Model file for the job. Use its own axes, mm. A direction names the side the tool comes from. Round coordinates to 2 decimals unless told otherwise and drop trailing zeros. Loops run counter-clockwise (first coordinate to the right, second up) from the corner with the lowest first, then second, coordinate; pieces in that order, holes last. Notation, with made-up numbers: M 33.5,28.25 L 83.5,28.25 A22 ccw 83.5,51.25 Z; hole C -27,56 d9. An arc over 180 degrees is marked long. Use a Markdown table: item, result. Add a question column.
Item 1: Tool access for faces 1 (the cylindrical face through (-40.561, 40.755, 0.01)), 2 (the conical face through (-39.694, -39.869, -0.418)), 3 (the conical face through (-39.694, 39.869, 0.418)), 4 (the cylindrical face through (39.512, 39.683, -0.005)): list every direction of +Z, -Z, +X, -X, +Y, -Y with a clear straight run to the whole face (end or side of a thin tool).
Item 2: Saw through at C-C on z = 0.05. Write the cut outline in (x, y).
Item 3: Wall check: L1, parallel to Y at x = 17.5, z = 0.2; L2, parallel to X at y = 34.5, z = -0.05. Give the ranges that are in metal, low to high. Write a range as from..to.
Item 4: Two-plate mould, pull along Y, no slides. Class faces 5 (the cylindrical face through (40.755, 40.561, 0.01)), 6 (the cylindrical face through (39.683, -39.512, -0.005)), 7 (the cylindrical face through (40.561, -40.755, 0.01)): +Y half, -Y half, draft (parallel to the pull), parting line (faces both ways), or undercut.
Item 5: Saw through at A-A on y = 9.5. Write the cut outline in (x, z), then the cut area to 3 significant figures.
Autodesk Inventor part; units mm, degrees
ref_plane "YZ Plane" through (0, 0, 0) normal (1, 0, 0) x (0, 1, 0)
ref_plane "XZ Plane" through (0, 0, 0) normal (0, 1, 0) x (-1, 0, 0)
ref_plane "XY Plane" through (0, 0, 0) normal (0, 0, 1) x (1, 0, 0)
sketch "Sketch1" plane through (0, 0, 0) normal (0, 0, 1) x (1, 0, 0)
  line L0 (0, 0) -> (0, 7.5) construction
  line L1 (10, 0) -> (0, 0) construction
  line L2 (0, 0) -> (-10, 0) construction
  line L3 (0, 0) -> (-31.8198, 31.8198) construction
  circle A0 centre (0, 0) radius 45 construction
  line L4 (0, 0) -> (0, 45) construction
  line L5 (-31.8198, 31.8198) -> (-31.8198, -24.2384) construction
  line L6 (-31.8198, -24.2384) -> (-31.8198, -31.8198) construction
  line L7 (-31.8198, 31.8198) -> (24.2384, 31.8198) construction
  line L8 (24.2384, 31.8198) -> (31.8198, 31.8198) construction
  line L9 (31.8198, 31.8198) -> (31.8198, -31.8198) construction
  line L10 (31.8198, -31.8198) -> (-31.8198, -31.8198) construction
  line L11 (0, 0) -> (39.9999, 0) construction
  line L12 (0, 0) -> (0, -40) construction
  line L13 (-31.8198, 44.3198) -> (0, 44.3198)
  line L14 (-44.3198, 31.8198) -> (-44.3198, 0)
  line L15 (-44.3198, 0) -> (0, 0) construction
  arc A1 (-31.8198, 44.3198) -> (-44.3198, 31.8198) centre (-31.8198, 31.8198) ccw
  point P0 (0, 50)
  dimension "d6" = 90
  dimension "d7" = 45
  dimension "d15" = 12.5
sketch "Sketch2" plane through (0, 0, 0) normal (1, 0, 0) x (0, 1, 0)
  line L0 (44.3198, 0) -> (44.3198, 0.75)
  line L1 (44.3198, 0.75) -> (42.8198, 0.3481)
  line L2 (42.8198, 0.3481) -> (42.8198, 0)
  line L3 (44.3198, 0) -> (42.8198, 0) construction
  line L4 (44.3198, 0) -> (44.3198, -0.75)
  line L5 (44.3198, -0.75) -> (42.8198, -0.3481)
  line L6 (42.8198, -0.3481) -> (42.8198, 0)
  dimension "d16" = 0.75
  dimension "d17" = 15
  dimension "d18" = 1.5
sweep "Sweep1" add profiles "Sketch2" path "Sketch1"
mirror "Mirror1" about plane through (0, 43.6835, 0) normal (1, 0, 0) of "Sweep1"
mirror "Mirror2" about plane through (-44.3198, 0, 0) normal (0, -1, 0) of "Sweep1", "Mirror1"
properties part number "Belt"
Entries:
| question | item | result |
|---|---|---|
| 1 | face 1 | +Z, -Z, -X, +Y |
| 1 | face 2 | -Z |
| 1 | face 3 | +Z |
| 1 | face 4 | +Z, -Z |
| 2 | outline | M -44.32,-31.82 A12.5 ccw -31.82,-44.32 L 31.82,-44.32 A12.5 ccw 44.32,-31.82 L 44.32,31.82 A12.5 ccw 31.82,44.32 L -31.82,44.32 A12.5 ccw -44.32,31.82 Z; hole M -42.82,-31.82 A11 ccw -31.82,-42.82 L 31.82,-42.82 A11 ccw 42.82,-31.82 L 42.82,31.82 A11 ccw 31.82,42.82 L -31.82,42.82 A11 ccw -42.82,31.82 Z |
| 3 | L1 | -44.32..-42.82, 42.82..44.32 |
| 3 | L2 | -44.03..-42.49, 42.49..44.03 |
| 4 | face 5 | +Y half |
| 4 | face 6 | undercut |
| 4 | face 7 | -Y half |
| 5 | outline | M -44.32,-0.75 L -42.82,-0.35 L -42.82,0.35 L -44.32,0.75 Z; M 42.82,-0.35 L 44.32,-0.75 L 44.32,0.75 L 42.82,0.35 Z |
| 5 | area | 3.29 mm2 |
